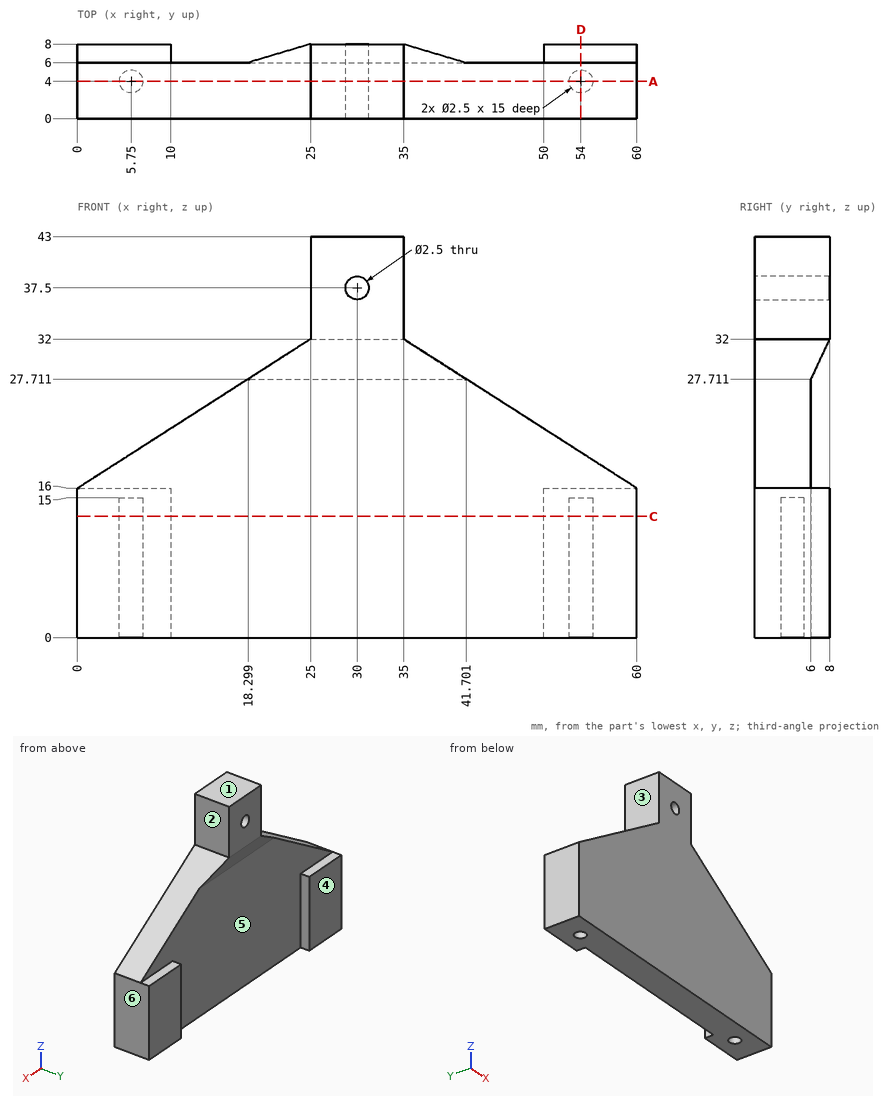
Input: dimensioned drawing with shaded views. Units: mm. Origin: part minimum x, y, z. A direction names the side the tool comes from. Give positions to 0.01 mm unless a question says otherwise; leave off trailing zeros. Loops run counter-clockwise (first coordinate to the right, second up) from the corner with the lowest first, then second, coordinate; pieces in that order, holes last. Notation, with made-up numbers: (48.5, -3) -> (86.5, -3) arc R19 cw to (86.5, 30) -> close; hole circle Ø3 at (38, 17). An arc over 180 degrees is marked (long way). Return JSON: item names as keys, results as strings.
Item 1: Line query: line 1 (Y direction, x = 54, z = 6.25); line 2 (X direction, y = 4.75, z = 37.5); line 3 (X direction, y = 1.5, z = 35.5). Output: solid intervals per line, ascending.
Filled in:
{"line 1": "0 to 2.75, 5.25 to 8", "line 2": "25 to 28.75, 31.25 to 35", "line 3": "25 to 35"}
Item 2: Section C-C, the plane z = 13. Output: boundary loops of the cut face in (x, y).
Filled in:
{"outline": "(0, 0) -> (60, 0) -> (60, 8) -> (50, 8) -> (50, 6) -> (10, 6) -> (10, 8) -> (0, 8) -> close; hole circle Ø2.5 at (5.75, 4); hole circle Ø2.5 at (54, 4)"}
Item 3: Section D-D, the plane x = 54. Output: boundary loops of the cut face in (y, z).
Filled in:
{"outline": "(0, 0) -> (2.75, 0) -> (2.75, 15) -> (5.25, 15) -> (5.25, 0) -> (8, 0) -> (8, 16) -> (6, 16) -> (6, 19.84) -> (0, 19.84) -> close"}
Item 4: Access query for the marked faces 1 and 2. Directions: +Z, -Z, +X, -X, +Y, -Y. A direction counts if a zero-diameter tool reaches every point of the face in a straight line with its end or side. Return the directions, or none.
Filled in:
{"face 1": "+Z, +X, -X, +Y, -Y", "face 2": "+Z, +X, +Y, -Y"}
Item 5: Mould query, pull axis X, two halves, no side actions, for the marked faces 3, 4, 5 and 6. Classes: released by +X, released by -X, zero draft, split by the parting line, or undercut.
Filled in:
{"face 3": "released by -X", "face 4": "zero draft", "face 5": "undercut", "face 6": "released by +X"}
Item 6: Section A-A, the plane y = 4. Output: boundary loops of the cut face in (x, z).
Filled in:
{"outline": "(0, 0) -> (4.5, 0) -> (4.5, 15) -> (7, 15) -> (7, 0) -> (52.75, 0) -> (52.75, 15) -> (55.25, 15) -> (55.25, 0) -> (60, 0) -> (60, 16) -> (35, 32) -> (35, 43) -> (25, 43) -> (25, 32) -> (0, 16) -> close; hole circle Ø2.5 at (30, 37.5)"}
Item 7: Pin query (flat end, axial travel): P1, Ø4, axis at y = 3.5, z = 36.5, coming from the -X side; P2, Ø1.6, axis at y = 7, z = 8.5, coming from the -X side; P3, Ø8.5, axis at x = 36.5, z = 11.5, coming from the +Y side; P4, Ø2, axis at x = 5.75, y = 4, coming from the -Z side. Return the tip coordinate at first contact, or that it passes through.
Filled in:
{"P1": "x = 25", "P2": "x = 0", "P3": "y = 6", "P4": "z = 15"}
